from build123d import *

# Parameters (mm, degrees)
BOSS_EXTRUDE1_DEPTH = 1.75
SKETCH2_R           = 7.5
BOSS_EXTRUDE2_DEPTH = 1.5
SKETCH3_R           = 1.95
CUT_EXTRUDE1_DEPTH  = 12.093353866
SKETCH4_R           = 0.8365
BOSS_EXTRUDE3_DEPTH = 1.5


with BuildPart() as part:
    # Sketch1 → Boss-Extrude1 (new body)
    with BuildSketch(Plane(origin=(0, 0, 0), x_dir=(1, 0, 0), z_dir=(0, 1, 0))):
        with BuildLine():
            Line((-2.616772822, 1.25), (2.616772822, 1.25))
            ThreePointArc((2.616772822, 1.25), (2.9, 0), (2.616772822, -1.25))
            Line((2.616772822, -1.25), (-2.616772822, -1.25))
            ThreePointArc((-2.616772822, -1.25), (-2.9, 0), (-2.616772822, 1.25))
        make_face()
    extrude(amount=BOSS_EXTRUDE1_DEPTH)

    # Sketch2 → Boss-Extrude2 (add)
    with BuildSketch(Plane(origin=(0, 1.75, 0), x_dir=(1, 0, 0), z_dir=(0, 1, 0))):
        with Locations(Location((0, 0, 0), (0, 0, 270))):
            Circle(SKETCH2_R)
    extrude(amount=BOSS_EXTRUDE2_DEPTH)

    # Sketch3 → Cut-Extrude1 (cut, through all)
    with BuildSketch(Plane(origin=(0, 3.25, 0), x_dir=(1, 0, 0), z_dir=(0, 1, 0))):
        with Locations(Location((0, 0, 0), (0, 0, 270))):
            Circle(SKETCH3_R)
    extrude(amount=-CUT_EXTRUDE1_DEPTH, mode=Mode.SUBTRACT)

    # Sketch4 → Boss-Extrude3 (add)
    with BuildSketch(Plane(origin=(0, 3.25, 0), x_dir=(1, 0, 0), z_dir=(0, 1, 0))):
        with Locations(Location((4, 4, 0), (0, 0, 270))):
            Circle(SKETCH4_R)
        with Locations(Location((-4, -4, 0), (0, 0, 270))):
            Circle(SKETCH4_R)
    extrude(amount=BOSS_EXTRUDE3_DEPTH)


solid = part.part
Work out the finished part from the listing and answer in its coordinate system (mm). A direction names the side the tool comes from. Coordinates: 2 decimals unless noted, no trailing zeros. Order: outer loops, then holes, each group sorted by start corner. A loop starts at its lowest first (then second) coordinate and runs counter-clockwise, first axis right, second up. Notation, with made-up numbers: (4.25, -3.5) - (53.25, -3.5) arc R17 ccw to (53.25, 20.5) - close; hole circle Ø10 at (71.25, 75.5). An arc over 180 degrees is marked (long way). Put each result on its own line as item: value. Start each with the question number.
1) For faces 1 (the cylindrical face through (-2.9, 0.9, 0)), 2 (the cylindrical face through (2.9, 0.9, 0)), 3 (the flat face through (-2, 1, -1.25)), 4 (the flat face through (-2, 1, 1.25)), 5 (the cylindrical face through (-4.32, 3.99, 4.773)), determine the directions among +Z, -Z, +X, -X, +Y, -Y from which every point of the face is accessible in a straight line to the end or side of a thin tool.
2) Flat-ended cylindrical pins translate along their axes: pin 1 (0.6 mm diameter, centred on x = 2.5, y = 1, fed in from -Z); pin 2 (7.5 mm diameter, centred on x = -2.5, z = 0, fed in from +Y); pin 3 (1 mm diameter, centred on x = -2.5, y = 2, fed in from -Z); pin 4 (2 mm diameter, centred on x = -2.5, y = 1, fed in from -Z). Find the tip coordinate at first contact, or state that the pin passes through.
3) For a pull along X with two mould halves and no side action, classify faces 6 (the flat face through (-2, 1.75, 2)), 7 (the cylindrical face through (4.565, 3.99, -4.617)), 8 (the cylindrical face through (-0.75, 2.01, 1.8)) as released by +X, released by -X, zero draft, split by the parting line, or undercut.
4) Find the intervals of material crossed by line 1 (Y direction, x = 2.75, z = -4); line 2 (Z direction, x = 4.75, y = 2.6); line 3 (Z direction, x = -3.75, y = 4.35), in increasing order. Write a range as from..to.
5) Find section D-D (y = 2.5). Give the vertices of the cut face in (x, z).
6) Find section C-C (z = 3.5). Give the vertices of the cut face in (x, y).
7) Find section A-A (y = 0.4). Give the vertices of the cut face in (x, z), plus the area to 3 significant figures.
8) Find section B-B (x = 0). Give the vertices of the cut face in (y, z), plus the area to 4 significant figures.
Results list:
1. face 1: -X, -Y
1. face 2: +X, -Y
1. face 3: -Z, +X, -X, -Y
1. face 4: +Z, +X, -X, -Y
1. face 5: +Y
2. pin 1: stops at z = -1.25
2. pin 2: stops at y = 4.75
2. pin 3: stops at z = -7.23
2. pin 4: stops at z = -7.27
3. face 6: zero draft
3. face 7: split by the parting line
3. face 8: undercut
4. line 1: y = 1.75..3.25
4. line 2: z = -5.8..5.8
4. line 3: z = 3.2..4.8
5. outline: circle Ø15 at (0, 0); hole circle Ø3.9 at (0, 0)
6. outline: (-6.63, 1.75) - (6.63, 1.75) - (6.63, 3.25) - (-3.33, 3.25) - (-3.33, 4.75) - (-4.67, 4.75) - (-4.67, 3.25) - (-6.63, 3.25) - close
7. outline: (-2.62, -1.25) - (-1.5, -1.25) arc R1.95 cw to (-1.5, 1.25) - (-2.62, 1.25) arc R2.9 ccw to start; (1.5, -1.25) - (2.62, -1.25) arc R2.9 ccw to (2.62, 1.25) - (1.5, 1.25) arc R1.95 cw to start
7. area: 5.00 mm^2
8. outline: (1.75, -7.5) - (3.25, -7.5) - (3.25, -1.95) - (1.75, -1.95) - close; (1.75, 1.95) - (3.25, 1.95) - (3.25, 7.5) - (1.75, 7.5) - close
8. area: 16.65 mm^2
